from build123d import *

# Parameters (mm, degrees)
SKETCH_1_W          = 43
SKETCH_1_H          = 80
EXTRUDE_1_DEPTH     = 9.5
CUT_EXTRUDE_1_DEPTH = 92.319494085
CHAMFER_1_SIZE      = 2.5
EXTRUDE_2_DEPTH     = 2
SKETCH_4_R          = 1.3
CUT_EXTRUDE_2_DEPTH = 92.549167118
SKETCH_5_R          = 2.15
CUT_EXTRUDE_3_DEPTH = 1.8
SKETCH_7_R          = 1.25
CUT_EXTRUDE_4_DEPTH = 5


with BuildPart() as part:
    # 草图1 → 凸台-拉伸1 (new body)
    with BuildSketch(Plane.XY):
        with Locations((21.5, -40)):
            Rectangle(SKETCH_1_W, SKETCH_1_H)
    extrude(amount=EXTRUDE_1_DEPTH)

    # 草图2 → 切除-拉伸1 (cut, through all)
    with BuildSketch(Plane(origin=(0, 0, 0), x_dir=(1, 0, 0), z_dir=(0, 1, 0))):
        Polygon((6.5, 0), (6.5, -1), (3.5, -4), (3.5, -7), (39.5, -7), (39.5, -4), (36.5, -1), (36.5, 0), align=None)
    extrude(amount=-CUT_EXTRUDE_1_DEPTH, mode=Mode.SUBTRACT)

    # 倒角1
    chamfer_1_edges = [part.edges().sort_by_distance(p)[0] for p in [
        (43, -40, 0),
        (0, -40, 0),
    ]]
    chamfer(chamfer_1_edges, length=CHAMFER_1_SIZE)

    # 草图3 → 凸台-拉伸2 (add)
    with BuildSketch(Plane.XY.offset(9.5)):
        with BuildLine():
            Line((17.5, -80), (25.5, -80))
            Line((25.5, -80), (25.5, -66))
            ThreePointArc((25.5, -66), (21.5, -62), (17.5, -66))
            Line((17.5, -66), (17.5, -80))
        make_face()
        with BuildLine():
            Line((17.5, -36), (17.5, 0))
            Line((17.5, 0), (25.5, 0))
            Line((25.5, 0), (25.5, -36))
            ThreePointArc((25.5, -36), (21.5, -40), (17.5, -36))
        make_face()
    extrude(amount=EXTRUDE_2_DEPTH)

    # 草图4 → 切除-拉伸2 (cut, through all)
    with BuildSketch(Plane.XY.offset(11.5)):
        with Locations((21.5, -36)):
            Circle(SKETCH_4_R)
        with Locations((21.5, -66)):
            Circle(SKETCH_4_R)
    extrude(amount=-CUT_EXTRUDE_2_DEPTH, mode=Mode.SUBTRACT)

    # 草图5 → 切除-拉伸3 (cut)
    with BuildSketch(Plane(origin=(0, 0, 7), x_dir=(-1, 0, 0), z_dir=(0, 0, -1))):
        with Locations((-21.5, -36)):
            Circle(SKETCH_5_R)
        with Locations((-21.5, -66)):
            Circle(SKETCH_5_R)
    extrude(amount=-CUT_EXTRUDE_3_DEPTH, mode=Mode.SUBTRACT)

    # 草图7 → 切除-拉伸4 (cut)
    with BuildSketch(Plane.ZY):
        with Locations(Location((5.2, -10, 0), (0, 0, 270))):
            Circle(SKETCH_7_R)
        with Locations(Location((5.2, -25, 0), (0, 0, 270))):
            Circle(SKETCH_7_R)
        with Locations(Location((5.2, -40, 0), (0, 0, 270))):
            Circle(SKETCH_7_R)
        with Locations(Location((5.2, -55, 0), (0, 0, 270))):
            Circle(SKETCH_7_R)
        with Locations(Location((5.2, -70, 0), (0, 0, 270))):
            Circle(SKETCH_7_R)
    extrude(amount=-CUT_EXTRUDE_4_DEPTH, mode=Mode.SUBTRACT)


solid = part.part
The listing builds one solid part. Answer for the finished solid, in the listing's coordinates (mm). A direction names the side the tool comes from. Coordinates: 2 decimals unless noted, no trailing zeros. Loops run counter-clockwise (first coordinate to the right, second up) from the corner with the lowest first, then second, coordinate; pieces in that order, holes last. Notation, with made-up numbers: (7, -10) -> (56, -10) arc R14 ccw to (56, 10) -> close; hole circle Ø5 at (23, 79.25). An arc over 180 degrees is marked (long way). Answer in a Markdown table with one row per item. Add a question column.
1. Consider line 1 (Y direction, x = 2.75, z = 5.2); line 2 (Y direction, x = 21.5, z = 7.4); line 3 (Z direction, x = 40, y = -22.5). Determine where each line is inside the solid, lowest interval first. Write a range as [from, to].
2. The part is cut by section A-A, the plane z = 10.5. Write down the section's boundary in (x, y), then the cut area to 3 significant figures.
3. The part is cut by section B-B, the plane z = 5.2. Write down the section's boundary in (x, y).
4. Determine the mould class of faces 4 (the flat face through (1.3, -40.6, 1.2)), 5 (the cylindrical face through (20.47, -66.79, 10.17)), 6 (the cylindrical face through (1.76, -26.19, 5.58)) for opening direction Z: +Z half, -Z half, draft (parallel to the pull), parting line (faces both ways), or undercut.
5. For faces 1 (the cylindrical face through (1.76, -56.19, 5.58)), 2 (the cylindrical face through (21.78, -33.87, 7.89)), 3 (the flat face through (21, -39, 7)), determine the directions among +Z, -Z, +X, -X, +Y, -Y from which every point of the face is accessible in a straight line to the end or side of a thin tool.
6. The part is cut by section D-D, the plane y = -46.5. Write down the section's boundary in (x, z).
7. The part is cut by section C-C, the plane x = 21.5. Write down the section's boundary in (y, z).
8. Flat-ended cylindrical pins translate along their axes: P1, Ø1.6, axis at y = -72.5, z = 10.5, coming from the -X side; P2, Ø1.3, axis at x = 22, y = -35, coming from the -Z side; P3, Ø7, axis at x = 21.5, y = -66, coming from the -Z side. Find the tip coordinate at first contact, or state that the pin passes through.
Answer below:
| question | item | result |
|---|---|---|
| 1 | line 1 | [-80, -71.25], [-68.75, -56.25], [-53.75, -41.25], [-38.75, -26.25], [-23.75, -11.25], [-8.75, 0] |
| 1 | line 2 | [-80, -68.15], [-63.85, -38.15], [-33.85, 0] |
| 1 | line 3 | [0, 9.5] |
| 2 | outline | (17.5, -80) -> (25.5, -80) -> (25.5, -66) arc R4 ccw to (17.5, -66) -> close; (17.5, -36) arc R4 ccw to (25.5, -36) -> (25.5, 0) -> (17.5, 0) -> close; hole circle Ø2.6 at (21.5, -66); hole circle Ø2.6 at (21.5, -36) |
| 2 | area | 440 mm2 |
| 3 | outline | (0, -80) -> (3.5, -80) -> (3.5, -71.25) -> (0, -71.25) -> close; (0, -68.75) -> (3.5, -68.75) -> (3.5, -56.25) -> (0, -56.25) -> close; (0, -53.75) -> (3.5, -53.75) -> (3.5, -41.25) -> (0, -41.25) -> close; (0, -38.75) -> (3.5, -38.75) -> (3.5, -26.25) -> (0, -26.25) -> close; (0, -23.75) -> (3.5, -23.75) -> (3.5, -11.25) -> (0, -11.25) -> close; (0, -8.75) -> (3.5, -8.75) -> (3.5, 0) -> (0, 0) -> close; (39.5, -80) -> (43, -80) -> (43, 0) -> (39.5, 0) -> close |
| 4 | face 4 | -Z half |
| 4 | face 5 | draft |
| 4 | face 6 | undercut |
| 5 | face 1 | -X |
| 5 | face 2 | -Z |
| 5 | face 3 | +Y, -Y |
| 6 | outline | (0, 2.5) -> (2.5, 0) -> (6.5, 0) -> (6.5, 1) -> (3.5, 4) -> (3.5, 7) -> (39.5, 7) -> (39.5, 4) -> (36.5, 1) -> (36.5, 0) -> (40.5, 0) -> (43, 2.5) -> (43, 9.5) -> (0, 9.5) -> close |
| 7 | outline | (-80, 7) -> (-68.15, 7) -> (-68.15, 8.8) -> (-67.3, 8.8) -> (-67.3, 11.5) -> (-80, 11.5) -> close; (-64.7, 8.8) -> (-63.85, 8.8) -> (-63.85, 7) -> (-38.15, 7) -> (-38.15, 8.8) -> (-37.3, 8.8) -> (-37.3, 11.5) -> (-40, 11.5) -> (-40, 9.5) -> (-62, 9.5) -> (-62, 11.5) -> (-64.7, 11.5) -> close; (-34.7, 8.8) -> (-33.85, 8.8) -> (-33.85, 7) -> (0, 7) -> (0, 11.5) -> (-34.7, 11.5) -> close |
| 8 | P1 | x = 17.5 |
| 8 | P2 | z = 8.8 |
| 8 | P3 | z = 7 |
